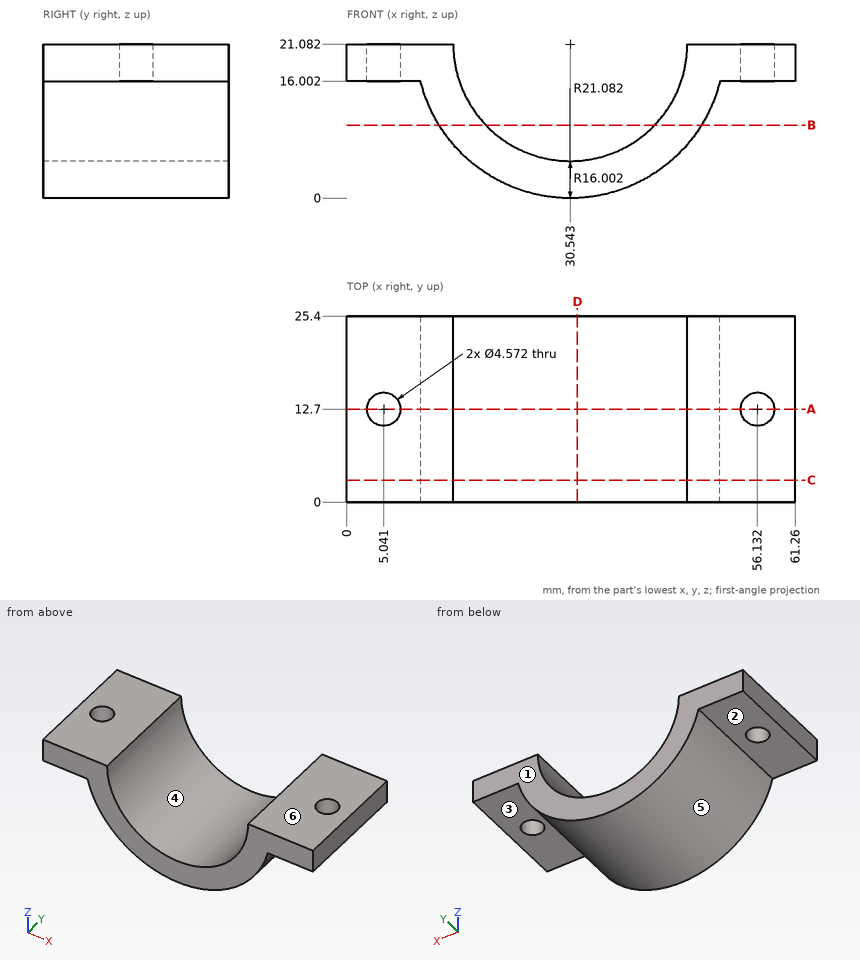
Part print with two shaded views. Sizes in mm from the minimum x, y, z corner. A direction names the side the tool comes from. Give positions to 0.01 mm unless a question says otherwise; leave off trailing zeros. Order: outer loops, then holes, each group sorted by start corner. A loop starts at its lowest first (then second) coordinate and runs counter-clockwise, first axis right, second up. Notation, with made-up numbers: M -39.75,-25.75 L -25.75,-25.75 A13 ccw -25.75,-21.75 Z; hole C -34,5 d8. An arc over 180 degrees is marked long. Write item = value, one per line.
Q1. Tool access for the marked faces 1, 2 and 3: list every direction of +Z, -Z, +X, -X, +Y, -Y with a clear straight run to the whole face (end or side of a thin tool).
Derived:
face_1 = +Z, -Z, +X, -X, +Y
face_2 = -Z, -X, +Y, -Y
face_3 = -Z, +X, +Y, -Y
Q2. Cut at B-B, the plane z = 10. List the corners of the cut face in (x, y).
Derived:
outline = M 12.61,0 L 19,0 L 19,25.4 L 12.61,25.4 Z; M 42.09,0 L 48.48,0 L 48.48,25.4 L 42.09,25.4 Z
Q3. Drill centre lines: line 1 (Z direction, x = 10, y = 6); line 2 (X direction, y = 9, z = 12.25) (1 decimal); line 3 (X direction, y = 19.5, z = 17.25). Where is each one in solid material? Low to high. Write a range as [from, to].
Derived:
line_1 = [16, 21.08]
line_2 = [11.4, 17.2], [43.9, 49.7]
line_3 = [0, 15.01], [46.08, 61.26]
Q4. Two-plate mould, pull along X, no slides. Class the marked faces 4, 5 and 6: pulls with the +X half, pulls with the -X half, needs draft (parallel to the pull), parting line crosses it, or undercut.
Derived:
face_4 = undercut
face_5 = parting line crosses it
face_6 = needs draft
Q5. Flat gauge pins, fed straight in: pin 1 (6 mm diameter, centred on y = 19, z = 2, fed in from +X) (1 decimal); pin 2 (8 mm diameter, centred on x = 6, y = 14, fed in from -Z); pin 3 (1.5 mm diameter, centred on x = 24, y = 6.5, fed in from +Z); pin 4 (2.5 mm diameter, centred on x = 56.13, y = 12.7, fed in from +Z). Where does each tip first touch, or does it go through?
Derived:
pin_1 = 44.2
pin_2 = 16
pin_3 = 6.84
pin_4 = through
Q6. Cut at A-A, the plane y = 12.7. List the corners of the cut face in (x, z) (1 decimal).
Derived:
outline = M 0,16 L 2.8,16 L 2.8,21.1 L 0,21.1 Z; M 7.3,16 L 10.1,16 A21.1 ccw 51,16 L 53.8,16 L 53.8,21.1 L 46.5,21.1 A16 cw 14.5,21.1 L 7.3,21.1 Z; M 58.4,16 L 61.3,16 L 61.3,21.1 L 58.4,21.1 Z
Q7. Cut at D-D, the plane x = 31.5. List the corners of the cut face in (y, z), then the cut area to 3 significant figures.
Derived:
outline = M 0,0.02 L 25.4,0.02 L 25.4,5.11 L 0,5.11 Z
area = 129 mm2
Q8. Cut at C-C, the plane y = 3. List the corners of the cut face in (x, z) (1 decimal).
Derived:
outline = M 0,16 L 10.1,16 A21.1 ccw 51,16 L 61.3,16 L 61.3,21.1 L 46.5,21.1 A16 cw 14.5,21.1 L 0,21.1 Z
